from build123d import *

# Parameters (mm, degrees)
SKETCH1_R           = 46
SKETCH1_R_2         = 3.5
BOSS_EXTRUDE1_DEPTH = 20
CHAMFER1_SIZE       = 1
SKETCH2_R           = 12
BOSS_EXTRUDE2_DEPTH = 10
SKETCH3_R           = 33
CUT_EXTRUDE1_DEPTH  = 14
SKETCH4_R           = 2.5
CUT_EXTRUDE2_DEPTH  = 6
SKETCH5_R           = 7
CUT_EXTRUDE3_DEPTH  = 10
CHAMFER2_SIZE       = 1
SKETCH6_R           = 4
CUT_EXTRUDE4_DEPTH  = 80


with BuildPart() as part:
    # Sketch1 → Boss-Extrude1 (new body)
    with BuildSketch(Plane.XY):
        Circle(SKETCH1_R)
        with Locations((0, 36)):
            Circle(SKETCH1_R_2, mode=Mode.SUBTRACT)
        with Locations((31.176914536, 18)):
            Circle(SKETCH1_R_2, mode=Mode.SUBTRACT)
        with Locations((31.176914536, -18)):
            Circle(SKETCH1_R_2, mode=Mode.SUBTRACT)
        with Locations((0, -36)):
            Circle(SKETCH1_R_2, mode=Mode.SUBTRACT)
        with Locations((-31.176914536, -18)):
            Circle(SKETCH1_R_2, mode=Mode.SUBTRACT)
        with Locations((-31.176914536, 18)):
            Circle(SKETCH1_R_2, mode=Mode.SUBTRACT)
    extrude(amount=BOSS_EXTRUDE1_DEPTH)

    # Chamfer1
    chamfer1_edges = [part.edges().sort_by_distance(p)[0] for p in [
        (-46, 0, 20),
    ]]
    chamfer(chamfer1_edges, length=CHAMFER1_SIZE)

    # Sketch2 → Boss-Extrude2 (add)
    with BuildSketch(Plane.XY.offset(20)):
        Circle(SKETCH2_R)
    extrude(amount=BOSS_EXTRUDE2_DEPTH)

    # Sketch3 → Cut-Extrude1 (cut)
    with BuildSketch(Plane(origin=(0, 0, 0), x_dir=(-1, 0, 0), z_dir=(0, 0, -1))):
        Circle(SKETCH3_R)
    extrude(amount=-CUT_EXTRUDE1_DEPTH, mode=Mode.SUBTRACT)

    # Sketch4 → Cut-Extrude2 (cut)
    with BuildSketch(Plane(origin=(0, 0, 14), x_dir=(-1, 0, 0), z_dir=(0, 0, -1))):
        Circle(SKETCH4_R)
    extrude(amount=-CUT_EXTRUDE2_DEPTH, mode=Mode.SUBTRACT)

    # Sketch5 → Cut-Extrude3 (cut)
    with BuildSketch(Plane.XY.offset(30)):
        Circle(SKETCH5_R)
    extrude(amount=-CUT_EXTRUDE3_DEPTH, mode=Mode.SUBTRACT)

    # Chamfer2
    chamfer2_edges = [part.edges().sort_by_distance(p)[0] for p in [
        (-7, 0, 30),
    ]]
    chamfer(chamfer2_edges, length=CHAMFER2_SIZE)

    # Sketch6 → Cut-Extrude4 (cut)
    with BuildSketch(Plane(origin=(0, 0, 0), x_dir=(0, 0, -1), z_dir=(1, 0, 0))):
        with Locations((-8, 0)):
            Circle(SKETCH6_R)
    extrude(amount=-CUT_EXTRUDE4_DEPTH, mode=Mode.SUBTRACT)


solid = part.part
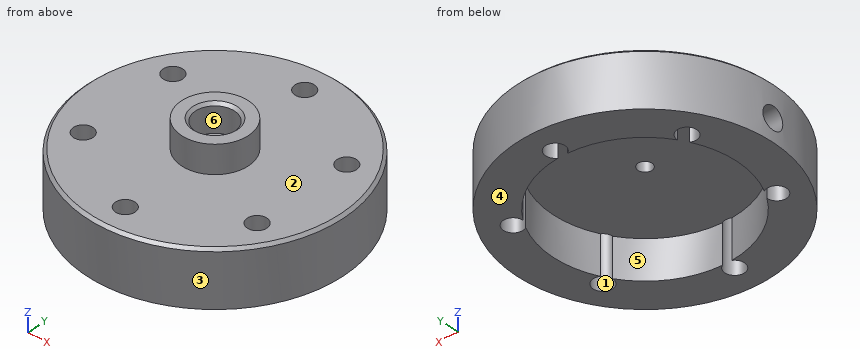
Could you check a few things on this model? Use its own coordinates, in mm. Face numbers are marked on the shaded views. A direction names the side the tool comes from. Give positions to 0.01 mm unless a question says otherwise; leave off trailing zeros. Order: outer loops, then holes, each group sorted by start corner. A loop starts at its lowest first (then second) coordinate and runs counter-clockwise, first axis right, second up.
1. Suppose I cut it at B-B (z = 10). Write out the boundary of the cut face in (x, y).
Answers below:
outline: (-45.87, -3.46) arc R46 ccw (long way) to (-45.87, 3.46) - (-32.82, 3.46) arc R33 cw to (-29.4, 14.98) arc R3.5 cw (long way) to (-27.68, 17.97) arc R33 cw to (-1.73, 32.95) arc R3.5 cw (long way) to (1.73, 32.95) arc R33 cw to (27.68, 17.97) arc R3.5 cw (long way) to (29.4, 14.98) arc R33 cw to (29.4, -14.98) arc R3.5 cw (long way) to (27.68, -17.97) arc R33 cw to (1.73, -32.95) arc R3.5 cw (long way) to (-1.73, -32.95) arc R33 cw to (-27.68, -17.97) arc R3.5 cw (long way) to (-29.4, -14.98) arc R33 cw to (-32.82, -3.46) - close
2. Which directions (+Z, -Z, +X, -X, +Y, -Y) give clear straight access to the entire face, cutting with the end or side of a thin tool? Please do the marked faces 4, 5 and 6.
Answers below:
face 4: -Z, +X, -X, +Y, -Y
face 5: -Z
face 6: +Z
3. Suppose I cut it at A-A (z = 17). Write out the boundary of the cut face in (x, y), plus the area to 3 significant figures.
Answers below:
outline: circle Ø92 at (0, 0); hole circle Ø7 at (-31.18, -18); hole circle Ø7 at (-31.18, 18); hole circle Ø7 at (0, -36); hole circle Ø7 at (0, 36); hole circle Ø5 at (0, 0); hole circle Ø7 at (31.18, -18); hole circle Ø7 at (31.18, 18)
area: 6,400 mm2
4. Thinking about a two-plate mould opening in X: for the marked faces 1, 2 and 3, which applies, +X half, -X half, draft (parallel to the pull), parting line (faces both ways), or undercut?
Answers below:
face 1: undercut
face 2: draft
face 3: parting line
5. Suppose I cut it at C-C (z = 25.5). Write out the boundary of the cut face in (x, y).
Answers below:
outline: circle Ø24 at (0, 0); hole circle Ø14 at (0, 0)
6. I need wall thicknesses on L1, parallel to Y at x = 1, z = 15.5; L2, parallel to Y at x = 0, z = 10.75; L3, parallel to Y at x = 2, z = 13.5. Which ranges of each line are inside material? Lowest first, please.
Answers below:
L1: y = -45.99 to -39.35, -32.65 to -2.29, 2.29 to 32.65, 39.35 to 45.99
L2: y = -46 to -39.5, 39.5 to 46
L3: y = -45.96 to -38.87, -33.13 to -32.94, 32.94 to 33.13, 38.87 to 45.96
7. For pin 1 (6.5 mm diameter, centred on x = 0, y = 0, fed in from +Z); pin 2 (2 mm diameter, centred on y = -5.5, z = 23.5, fed in from +X); pin 3 (20 mm diameter, centred on x = -4.5, y = -3.5, fed in from -Z); pin 4 (6.5 mm diameter, centred on x = 31.18, y = 18, fed in from +Z), each with a flat end and sliding along its axis, tell me the tip position at first contact or that it passes through.
Answers below:
pin 1: stops at z = 20
pin 2: stops at x = 11.12
pin 3: stops at z = 14
pin 4: passes through
